Part model, mm, in its own coordinate system. Give positions to 0.01 mm unless a question says otherwise; leave off trailing zeros. Write each loop counter-clockwise with the first axis right and the second up, starting at its lowest first coordinate (ties: lowest second). Pieces come first, ordered by that corner, then holes.
```python
from build123d import *

# Parameters (mm, degrees)
SKETCH_1_W               = 93
SKETCH_1_H               = 60
EXTRUDE_1_DEPTH          = 1.5
SKETCH_2_R               = 21.75
CUT_EXTRUDE_1_DEPTH      = 12
SKETCH_3_R               = 1.275
CUT_EXTRUDE_2_DEPTH      = 12
SKETCH_4_R               = 1.525
CUT_EXTRUDE_3_DEPTH      = 15
CUT_EXTRUDE_5_DEPTH      = 10
FILLET_1_R               = 2
CUT_EXTRUDE_6_DEPTH      = 10
FILLET_2_R               = 2
SKETCH_10_W              = 16
SKETCH_10_H              = 6
EXTRUDE_2_DEPTH          = 3
MIRROR_5_COPY_1_SKETCH_W = 16
MIRROR_5_COPY_1_SKETCH_H = 6
MIRROR_5_COPY_1_DEPTH    = 3
SKETCH_11_R              = 1.025
CUT_EXTRUDE_8_DEPTH      = 3


with BuildPart() as part:
    # 草图1 → 凸台-拉伸1 (new body, symmetric)
    with BuildSketch(Plane.XY):
        Rectangle(SKETCH_1_W, SKETCH_1_H)
    extrude(amount=EXTRUDE_1_DEPTH, both=True)

    # 草图2 → 切除-拉伸1 (cut, symmetric)
    with BuildSketch(Plane.XY.offset(1.5)):
        Circle(SKETCH_2_R)
    extrude(amount=CUT_EXTRUDE_1_DEPTH, both=True, mode=Mode.SUBTRACT)

    # 草图3 → 切除-拉伸2 (cut, symmetric)
    with BuildSketch(Plane.XY.offset(1.5)):
        with Locations((21.217622393, 12.25)):
            Circle(SKETCH_3_R)
        with Locations((21.217622393, -12.25)):
            Circle(SKETCH_3_R)
        with Locations((0, -24.5)):
            Circle(SKETCH_3_R)
        with Locations((-21.217622393, -12.25)):
            Circle(SKETCH_3_R)
        with Locations((-21.217622393, 12.25)):
            Circle(SKETCH_3_R)
        with Locations((0, 24.5)):
            Circle(SKETCH_3_R)
    extrude(amount=CUT_EXTRUDE_2_DEPTH, both=True, mode=Mode.SUBTRACT)

    # 草图4 → 切除-拉伸3 (cut, symmetric)
    with BuildSketch(Plane.XY.offset(1.5)):
        with Locations((40.5, -22)):
            Circle(SKETCH_4_R)
        with Locations((40.5, 22)):
            Circle(SKETCH_4_R)
        with Locations((-40.5, -22)):
            Circle(SKETCH_4_R)
        with Locations((-40.5, 22)):
            Circle(SKETCH_4_R)
    extrude(amount=CUT_EXTRUDE_3_DEPTH, both=True, mode=Mode.SUBTRACT)

    # 草图6 → 切除-拉伸5 (cut)
    with BuildSketch(Plane.XY.offset(1.5)):
        with BuildLine():
            Line((26.355760449, 11.48635674), (41.5, 19.14393604))
            Line((41.5, 19.14393604), (41.5, -19.14393604))
            Line((41.5, -19.14393604), (26.355760449, -11.48635674))
            ThreePointArc((26.355760449, -11.48635674), (28.75, 0), (26.355760449, 11.48635674))
        make_face()
    cut_extrude_5 = extrude(amount=-CUT_EXTRUDE_5_DEPTH, mode=Mode.SUBTRACT)

    # 镜向1: 切除-拉伸5 across plane
    add(cut_extrude_5.mirror(Plane(origin=(0, 0, 0), x_dir=(0, 0, 1), z_dir=(1, 0, 0))), mode=Mode.SUBTRACT)

    # 圆角1
    fillet_1_edges = [part.edges().sort_by_distance(p)[0] for p in [
        (-26.355760449, 11.48635674, 0),
        (-26.355760449, -11.48635674, 0),
        (-41.5, -19.14393604, 0),
        (-41.5, 19.14393604, 0),
        (46.5, -30, 0),
        (-46.5, -30, 0),
        (-46.5, 30, 0),
        (46.5, 30, 0),
        (26.355760449, -11.48635674, 0),
        (26.355760449, 11.48635674, 0),
        (41.5, 19.14393604, 0),
        (41.5, -19.14393604, 0),
    ]]
    fillet(fillet_1_edges, radius=FILLET_1_R)

    # 草图8 → 切除-拉伸6 (cut)
    with BuildSketch(Plane.XY.offset(1.5)):
        with BuildLine():
            Line((14.197270865, 25), (39.784659393, 25))
            Line((39.784659393, 25), (23.393786426, 16.712069192))
            ThreePointArc((23.393786426, 16.712069192), (19.246930829, 21.356922851), (14.197270865, 25))
        make_face()
        with BuildLine():
            Line((39.784659393, -25), (23.393786426, -16.712069192))
            ThreePointArc((23.393786426, -16.712069192), (19.246930829, -21.356922851), (14.197270865, -25))
            Line((14.197270865, -25), (39.784659393, -25))
        make_face()
    cut_extrude_6 = extrude(amount=-CUT_EXTRUDE_6_DEPTH, mode=Mode.SUBTRACT)

    # 镜向2: 切除-拉伸6 across plane
    add(cut_extrude_6.mirror(Plane(origin=(0, 0, 0), x_dir=(0, 0, 1), z_dir=(1, 0, 0))), mode=Mode.SUBTRACT)

    # 圆角2
    fillet_2_edges = [part.edges().sort_by_distance(p)[0] for p in [
        (23.393786426, 16.712069192, 0),
        (14.197270865, 25, 0),
        (39.784659393, 25, 0),
        (14.197270865, -25, 0),
        (23.393786426, -16.712069192, 0),
        (39.784659393, -25, 0),
        (-14.197270865, 25, 0),
        (-23.393786426, 16.712069192, 0),
        (-39.784659393, 25, 0),
        (-23.393786426, -16.712069192, 0),
        (-14.197270865, -25, 0),
        (-39.784659393, -25, 0),
    ]]
    fillet(fillet_2_edges, radius=FILLET_2_R)

    # 草图10 → 凸台-拉伸2 (add)
    with BuildSketch(Plane(origin=(0, 0, -1.5), x_dir=(-1, 0, 0), z_dir=(0, 0, -1))):
        with Locations((-24.5, 30)):
            Rectangle(SKETCH_10_W, SKETCH_10_H)
    extrude_2 = extrude(amount=-EXTRUDE_2_DEPTH)

    # 镜向4: 凸台-拉伸2 across plane
    add(extrude_2.mirror(Plane(origin=(0, 0, 0), x_dir=(0, 0, 1), z_dir=(1, 0, 0))))

    # 镜向5: 凸台-拉伸2 across plane
    add(extrude_2.mirror(Plane.ZX))

    # 镜向5 copy 1 sketch → 镜向5 copy 1 (add)
    with BuildSketch(Plane(origin=(0, 0, -1.5), x_dir=(1, 0, 0), z_dir=(0, 0, -1))):
        with Locations((-24.5, 30)):
            Rectangle(MIRROR_5_COPY_1_SKETCH_W, MIRROR_5_COPY_1_SKETCH_H)
    extrude(amount=-MIRROR_5_COPY_1_DEPTH)

    # 草图11 → 切除-拉伸8 (cut)
    with BuildSketch(Plane.XY.offset(1.5)):
        with Locations((33.525, 30)):
            Circle(SKETCH_11_R)
        with Locations((15.475, 30)):
            Circle(SKETCH_11_R)
        with Locations((-15.475, 30)):
            Circle(SKETCH_11_R)
        with Locations((-33.525, 30)):
            Circle(SKETCH_11_R)
        with Locations((-33.525, -30)):
            Circle(SKETCH_11_R)
        with Locations((-15.475, -30)):
            Circle(SKETCH_11_R)
        with Locations((15.475, -30)):
            Circle(SKETCH_11_R)
        with Locations((33.525, -30)):
            Circle(SKETCH_11_R)
    extrude(amount=-CUT_EXTRUDE_8_DEPTH, mode=Mode.SUBTRACT)


solid = part.part
```
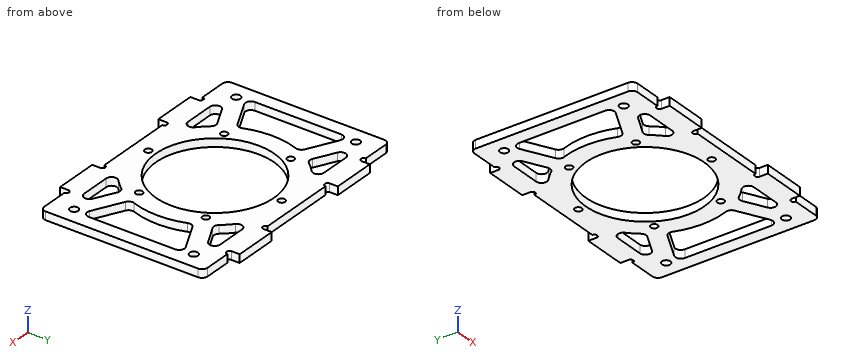
1) Saw through at D-D, the plane x = -23.5. Write the cut outline in (y, z), then the cut area to 3 significant figures.
Answers follow:
outline: (-33, -1.5) - (-25, -1.5) - (-25, 1.5) - (-33, 1.5) - close; (-17.31, -1.5) - (17.31, -1.5) - (17.31, 1.5) - (-17.31, 1.5) - close; (25, -1.5) - (33, -1.5) - (33, 1.5) - (25, 1.5) - close
area: 152 mm2
2) Wall check: L1, parallel to Y at x = 0, z = -0.45 (3 decimals); L2, parallel to X at y = -7.5, z = 0.2; L3, parallel to Y at x = -40.5, z = -0.8 (3 decimals). Give the ranges that are in metal, low to high.
Answers follow:
L1: y = -30 to -25.775, -23.225 to -21.75, 21.75 to 23.225, 25.775 to 30
L2: x = -46.5 to -41.5, -27.75 to -20.42, 20.42 to 27.75, 41.5 to 46.5
L3: y = -30 to -23.525, -20.475 to -17.624, 17.624 to 20.475, 23.525 to 30
3) Saw through at B-B, the plane y = -2. Write the cut outline in (x, z).
Answers follow:
outline: (-46.5, -1.5) - (-41.5, -1.5) - (-41.5, 1.5) - (-46.5, 1.5) - close; (-28.68, -1.5) - (-21.66, -1.5) - (-21.66, 1.5) - (-28.68, 1.5) - close; (21.66, -1.5) - (28.68, -1.5) - (28.68, 1.5) - (21.66, 1.5) - close; (41.5, -1.5) - (46.5, -1.5) - (46.5, 1.5) - (41.5, 1.5) - close
4) Pin check, flat tips, straight feed: pin 1 Ø0.9 at (x, z) = (38, 0.5) entering from +Y; pin 2 Ø2 at (x, y) = (-21.22, -12.25) entering from +Z; pin 3 Ø0.9 at (y, z) = (-31, 0.5) entering from -X. Stop position of each tip, or through.
Answers follow:
pin 1: stops at y = 30
pin 2: passes through
pin 3: stops at x = -32.5
5) Saw through at C-C, the plane z = -0.4. Count the separate pieces of the cut face and the enclosed holes in it, then the cut area to 3 significant figures.
Answers follow:
separate pieces: 1
enclosed holes: 17
area: 3,040 mm2
6) Saw through at A-A, the plane x = 5. Write the cut outline in (y, z).
Answers follow:
outline: (-30, -1.5) - (-21.17, -1.5) - (-21.17, 1.5) - (-30, 1.5) - close; (21.17, -1.5) - (30, -1.5) - (30, 1.5) - (21.17, 1.5) - close
